from build123d import *

# Parameters (mm, degrees)
AL_I_BEAM_AL_I_BEAM_4X2_31_4_DEPTH = 914.4
F_3_8_CLEARANCE_HOLE1_REACH        = 476.511
F_3_8_CLEARANCE_HOLE1_BORE_R       = 5.0419
F_1_2_CLEARANCE_HOLE1_D            = 13.49248
F_1_2_CLEARANCE_HOLE1_DEPTH        = 5.842


with BuildPart() as part:
    # Sketch11 → Al i beam AL I BEAM 4X2.31(4) (new body)
    with BuildSketch(Plane(origin=(53.975, -457.2, -38.1), x_dir=(0, 0, -1), z_dir=(0, 1, 0))):
        with BuildLine():
            Line((-38.1, -50.8), (-38.1, -44.958))
            Line((-38.1, -44.958), (-8.255, -44.958))
            ThreePointArc((-8.255, -44.958), (-3.764871939, -43.098128061), (-1.905, -38.608))
            Line((-1.905, -38.608), (-1.905, 38.608))
            ThreePointArc((-1.905, 38.608), (-3.764871939, 43.098128061), (-8.255, 44.958))
            Line((-8.255, 44.958), (-38.1, 44.958))
            Line((-38.1, 44.958), (-38.1, 50.8))
            Line((-38.1, 50.8), (38.1, 50.8))
            Line((38.1, 50.8), (38.1, 44.958))
            Line((38.1, 44.958), (8.255, 44.958))
            ThreePointArc((8.255, 44.958), (3.764871939, 43.098128061), (1.905, 38.608))
            Line((1.905, 38.608), (1.905, -38.608))
            ThreePointArc((1.905, -38.608), (3.764871939, -43.098128061), (8.255, -44.958))
            Line((8.255, -44.958), (38.1, -44.958))
            Line((38.1, -44.958), (38.1, -50.8))
            Line((38.1, -50.8), (-38.1, -50.8))
        make_face()
    extrude(amount=AL_I_BEAM_AL_I_BEAM_4X2_31_4_DEPTH)

    # 3/8 Clearance Hole1 bore → 3/8 Clearance Hole1 (cut, up to next)
    with BuildSketch(Plane(origin=(3.175, 0, 0), x_dir=(0, 0, -1), z_dir=(-1, 0, 0)), mode=Mode.PRIVATE) as f_3_8_clearance_hole1_sk1:
        with Locations((14.9225, -326.571428209)):
            Circle(F_3_8_CLEARANCE_HOLE1_BORE_R)
    f_3_8_clearance_hole1_tool1 = extrude(f_3_8_clearance_hole1_sk1.sketch, amount=-F_3_8_CLEARANCE_HOLE1_REACH, mode=Mode.PRIVATE) & part.part
    # 3/8 Clearance Hole1 bore → 3/8 Clearance Hole1 (cut, up to next)
    with BuildSketch(Plane(origin=(3.175, 0, 0), x_dir=(0, 0, -1), z_dir=(-1, 0, 0)), mode=Mode.PRIVATE) as f_3_8_clearance_hole1_sk2:
        with Locations((14.9225, 326.571428571)):
            Circle(F_3_8_CLEARANCE_HOLE1_BORE_R)
    f_3_8_clearance_hole1_tool2 = extrude(f_3_8_clearance_hole1_sk2.sketch, amount=-F_3_8_CLEARANCE_HOLE1_REACH, mode=Mode.PRIVATE) & part.part
    # 3/8 Clearance Hole1 bore → 3/8 Clearance Hole1 (cut, up to next)
    with BuildSketch(Plane(origin=(3.175, 0, 0), x_dir=(0, 0, -1), z_dir=(-1, 0, 0)), mode=Mode.PRIVATE) as f_3_8_clearance_hole1_sk3:
        with Locations((14.9225, 195.942857215)):
            Circle(F_3_8_CLEARANCE_HOLE1_BORE_R)
    f_3_8_clearance_hole1_tool3 = extrude(f_3_8_clearance_hole1_sk3.sketch, amount=-F_3_8_CLEARANCE_HOLE1_REACH, mode=Mode.PRIVATE) & part.part
    # 3/8 Clearance Hole1 bore → 3/8 Clearance Hole1 (cut, up to next)
    with BuildSketch(Plane(origin=(3.175, 0, 0), x_dir=(0, 0, -1), z_dir=(-1, 0, 0)), mode=Mode.PRIVATE) as f_3_8_clearance_hole1_sk4:
        with Locations((14.9225, 65.314285859)):
            Circle(F_3_8_CLEARANCE_HOLE1_BORE_R)
    f_3_8_clearance_hole1_tool4 = extrude(f_3_8_clearance_hole1_sk4.sketch, amount=-F_3_8_CLEARANCE_HOLE1_REACH, mode=Mode.PRIVATE) & part.part
    # 3/8 Clearance Hole1 bore → 3/8 Clearance Hole1 (cut, up to next)
    with BuildSketch(Plane(origin=(3.175, 0, 0), x_dir=(0, 0, -1), z_dir=(-1, 0, 0)), mode=Mode.PRIVATE) as f_3_8_clearance_hole1_sk5:
        with Locations((14.9225, -65.314285497)):
            Circle(F_3_8_CLEARANCE_HOLE1_BORE_R)
    f_3_8_clearance_hole1_tool5 = extrude(f_3_8_clearance_hole1_sk5.sketch, amount=-F_3_8_CLEARANCE_HOLE1_REACH, mode=Mode.PRIVATE) & part.part
    # 3/8 Clearance Hole1 bore → 3/8 Clearance Hole1 (cut, up to next)
    with BuildSketch(Plane(origin=(3.175, 0, 0), x_dir=(0, 0, -1), z_dir=(-1, 0, 0)), mode=Mode.PRIVATE) as f_3_8_clearance_hole1_sk6:
        with Locations((14.9225, -195.942856853)):
            Circle(F_3_8_CLEARANCE_HOLE1_BORE_R)
    f_3_8_clearance_hole1_tool6 = extrude(f_3_8_clearance_hole1_sk6.sketch, amount=-F_3_8_CLEARANCE_HOLE1_REACH, mode=Mode.PRIVATE) & part.part
    add(f_3_8_clearance_hole1_tool1.solids().sort_by_distance((3.175, 326.571428, -14.9225))[0], mode=Mode.SUBTRACT)
    add(f_3_8_clearance_hole1_tool2.solids().sort_by_distance((3.175, -326.571429, -14.9225))[0], mode=Mode.SUBTRACT)
    add(f_3_8_clearance_hole1_tool3.solids().sort_by_distance((3.175, -195.942857, -14.9225))[0], mode=Mode.SUBTRACT)
    add(f_3_8_clearance_hole1_tool4.solids().sort_by_distance((3.175, -65.314286, -14.9225))[0], mode=Mode.SUBTRACT)
    add(f_3_8_clearance_hole1_tool5.solids().sort_by_distance((3.175, 65.314285, -14.9225))[0], mode=Mode.SUBTRACT)
    add(f_3_8_clearance_hole1_tool6.solids().sort_by_distance((3.175, 195.942857, -14.9225))[0], mode=Mode.SUBTRACT)

    # 1/2 Clearance Hole1
    with Locations(Plane.ZY.offset(-98.933)):
        with Locations((-14.9225, 304.8), (-14.9225, -304.8), (-14.9225, -152.4), (-14.9225, 0), (-14.9225, 152.4)):
            Hole(F_1_2_CLEARANCE_HOLE1_D / 2, depth=F_1_2_CLEARANCE_HOLE1_DEPTH)


solid = part.part
Read the model definition and answer for the solid it produces. Units are mm, in the model's axes. A direction names the side the tool comes from. Give positions to 0.01 mm unless a question says otherwise; leave off trailing zeros. Write each loop counter-clockwise with the first axis right and the second up, starting at its lowest first coordinate (ties: lowest second). Pieces come first, ordered by that corner, then holes. Notation, with made-up numbers: (84, 49) - (120, 49) arc R8 ccw to (120, 56) - close; hole circle Ø9 at (7.25, 54). An arc over 180 degrees is marked (long way). Use CSV: the item, a comma, the result in double quotes. Start each with the question number.
(1) For faces 1 (the flat face through (9.017, -6, -15)), 2 (the flat face through (104.775, -6, -39)), 3 (the flat face through (9.017, -6, -61)), determine the directions among +Z, -Z, +X, -X, +Y, -Y from which every point of the face is accessible in a straight line to the end or side of a thin tool.
(2) Find section A-A (x = 38). Give the vertices of the cut face in (y, z) (3 decimals).
(3) Given P1, Ø10, axis at x = 43.5, y = -269.5, coming from the +Z side (3 decimals); P2, Ø8, axis at y = -195.94, z = -14.92, coming from the -X side; P3, Ø8, axis at x = 90.5, y = 265.5, coming from the -Z side, each flat-ended and moving along its own axis, determine where each tip first touches the part or whether it passes through.
(4) Determine the mould class of faces 4 (the flat face through (46, -457.2, -38)), 5 (the flat face through (55, -6, -36.195)), 6 (the flat face through (46, 457.2, -38)) for opening direction Y: +Y half, -Y half, draft (parallel to the pull), parting line (faces both ways), or undercut.
(5) Consider line 1 along X through (y, z) = (-128, -53) (3 decimals); line 2 along Z through (x, y) = (102, 304); line 3 along Z through (x, y) = (100, 152). Determine where each line is inside the solid, lowest interval first.
Findings below:
1,face 1,"+Z, +Y, -Y"
1,face 2,"+Z, -Z, +X, +Y, -Y"
1,face 3,"-Z, +Y, -Y"
2,outline,"(-457.2, -40.005) - (457.2, -40.005) - (457.2, -36.195) - (-457.2, -36.195) - close"
3,P1,"z = -36.195"
3,P2,"x = 98.93"
3,P3,"z = -40.3"
4,face 4,"-Y half"
4,face 5,"draft"
4,face 6,"+Y half"
5,line 1,"3.175 to 9.017, 98.933 to 104.775"
5,line 2,"-76.2 to -21.62, -8.22 to 0"
5,line 3,"-76.2 to -21.66, -8.19 to 0"
